Check sheet for the modelled part. Datum: model origin and axes. Units: mm. Coordinates: 2 decimals unless noted, no trailing zeros. Loops run counter-clockwise (first coordinate to the right, second up) from the corner with the lowest first, then second, coordinate; pieces in that order, holes last.
```python
from build123d import *

# Parameters (mm, degrees)
F0_R          = 38.1
F1_DEPTH      = 6.35
F2_R          = 12.7
F3_DEPTH      = 25.4
F8_R          = 1.27
F9_DEPTH      = 51.9166590996
F9_DEPTH_BACK = 51.9166590996


with BuildPart() as f1:
    # F0 (on Front) → F1 (new body, symmetric)
    with BuildSketch(Plane.XZ):
        Circle(F0_R)
    extrude(amount=F1_DEPTH, both=True)

    # F2 (on face) → F3 (cut)
    with BuildSketch(Plane.XZ.offset(6.35)):
        Circle(F2_R)
    extrude(amount=-F3_DEPTH, mode=Mode.SUBTRACT)

    # F8 (on face) → F9 (cut, two sides)
    with BuildSketch(Plane(origin=(0, 0, 0), x_dir=(0.8756408079, -0.1427525977, 0.4613836487), z_dir=(-0.4829629131, -0.2588190451, 0.8365163037))) as f9_sk:
        with Locations((25.4, 0)):
            Circle(F8_R)
    extrude(amount=-F9_DEPTH, mode=Mode.SUBTRACT)
    extrude(f9_sk.sketch, amount=F9_DEPTH_BACK, mode=Mode.SUBTRACT)


solid = f1.part
```
1) Section check C-C on x = -11. Enter the section's corners in (y, z), plus the area to 3 significant figures.
Answer sheet:
outline: (-6.35, -36.48) - (6.35, -36.48) - (6.35, -6.35) - (-6.35, -6.35) - close; (-6.35, 6.35) - (6.35, 6.35) - (6.35, 36.48) - (-6.35, 36.48) - close
area: 765 mm2
2) Mould release check, pull along Z, two halves, no side actions. Record for faces 1 (the flat face through (16, 6.35, 1)), 2 (the cylindrical face through (-2.75, -0.09, -12.4)), 3 (the cylindrical face through (-30.235, -0.089, -23.183)): +Z half, -Z half, draft (parallel to the pull), parting line (faces both ways), or undercut.
Answer sheet:
face 1: draft
face 2: undercut
face 3: parting line
3) Scan lines: line 1 (Z direction, x = 0, y = -2); line 2 (X direction, y = 4.75, z = -0.5); line 3 (X direction, y = -3.5, z = 5). Record each from-to range of solid material in increasing order.
Answer sheet:
line 1: z = -38.1 to -12.7, 12.7 to 38.1
line 2: x = -38.1 to -12.69, 12.69 to 38.1
line 3: x = -37.77 to -11.67, 11.67 to 37.77
4) Depth check by flat-ended pin: pin 1 (23 mm diameter, centred on x = 0, z = 0, fed in from +Y); pin 2 (4 mm diameter, centred on y = -5, z = 22, fed in from -X); pin 3 (6 mm diameter, centred on y = -3, z = 22.5, fed in from +X); pin 4 (5 mm diameter, centred on x = -29, y = -3.5, fed in from -Z). Enter the tip coordinate at first touch or a pass-through.
Answer sheet:
pin 1: passes through
pin 2: stops at x = -32.43
pin 3: stops at x = 32.73
pin 4: stops at z = -27.37
5) Section check B-B on z = 0. Give the number of separate pieces and of enclosed holes in the cut face, plus the area to 3 significant figures.
Answer sheet:
separate pieces: 2
enclosed holes: 1
area: 639 mm2
6) Section check D-D on z = 31. Enter the section's corners in (x, y).
Answer sheet:
outline: (-22.15, -6.35) - (22.15, -6.35) - (22.15, 6.35) - (-22.15, 6.35) - close
7) Section check A-A on x = 0. Enter the section's corners in (y, z), plus the area to 3 significant figures.
Answer sheet:
outline: (-6.35, -38.1) - (6.35, -38.1) - (6.35, -12.7) - (-6.35, -12.7) - close; (-6.35, 12.7) - (6.35, 12.7) - (6.35, 38.1) - (-6.35, 38.1) - close
area: 645 mm2
